Geometry: see drawing. Coordinates: mm, zero at the bounding-box minimum. Coordinates: 2 decimals unless noted, no trailing zeros. Write each loop counter-clockwise with the first axis right and the second up, starting at its lowest first coordinate (ties: lowest second). Pieces come first, ordered by that corner, then holes. Notation, with made-up numbers: M 48,29.25 L 104,29.25 A19 ccw 104,40.25 Z; hole C 53,-37 d10. An arc over 180 degrees is marked long. Answer as CSV lines item,"result". Start each with the question number.
1. Line query: probe 1 along X at (y, z) = (34, 1.1). Output: solid intervals per line, ascending. Write a range as [from, to].
2. Section B-B on y = 59. Return the cut outline in (x, z).
3. Contact query for flat-ended pins moving along their axis: pin 1 Ø1.4 at (x, z) = (157.5, 2.5) entering from +Y (1 decimal); pin 2 Ø1.4 at (y, z) = (15, 1.5) entering from +X; pin 3 Ø2.5 at (x, z) = (2.5, 3) entering from -Y. Output: stop coordinate, or through.
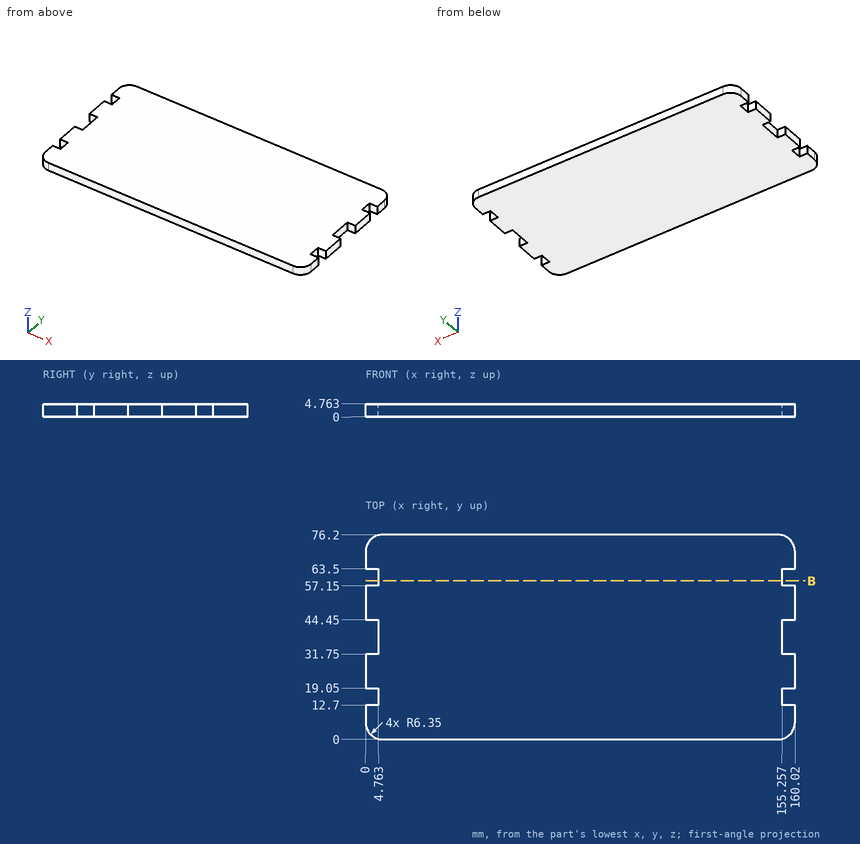
Values:
1,probe 1,"[4.76, 155.26]"
2,outline,"M 4.76,0 L 155.26,0 L 155.26,4.76 L 4.76,4.76 Z"
3,pin 1,"y = 75.4"
3,pin 2,"x = 155.26"
3,pin 3,"y = 0.56"
